```python
from build123d import *

# Parameters (mm, degrees)
ESQUISSE1_W          = 40
ESQUISSE1_H          = 60
PCB_RFID_RC522_DEPTH = 2
ANTENNE_RFID_START   = 2
ESQUISSE2_W          = 30
ESQUISSE2_H          = 32
ESQUISSE2_W_2        = 22
ESQUISSE2_H_2        = 24
ANTENNE_RFID_DEPTH   = 1.2
PUCE_MFRC522_START   = 2
ESQUISSE3_W          = 10
ESQUISSE3_H          = 10
PUCE_MFRC522_DEPTH   = 2.5
ESQUISSE4_W          = 22
ESQUISSE4_H          = 3
CONNECTEUR_SPI_DEPTH = 5


with BuildPart() as part:
    # Esquisse1 → PCB_RFID_RC522 (new body)
    with BuildSketch(Plane.XY):
        Rectangle(ESQUISSE1_W, ESQUISSE1_H)
    extrude(amount=PCB_RFID_RC522_DEPTH)

    # Esquisse2 → Antenne_RFID (add)
    with BuildSketch(Plane.XY.offset(ANTENNE_RFID_START)):
        with Locations((0, 8)):
            Rectangle(ESQUISSE2_W, ESQUISSE2_H)
        with Locations((0, 8)):
            Rectangle(ESQUISSE2_W_2, ESQUISSE2_H_2, mode=Mode.SUBTRACT)
    extrude(amount=ANTENNE_RFID_DEPTH)

    # Esquisse3 → Puce_MFRC522 (add)
    with BuildSketch(Plane.XY.offset(PUCE_MFRC522_START)):
        with Locations((0, -15)):
            Rectangle(ESQUISSE3_W, ESQUISSE3_H)
    extrude(amount=PUCE_MFRC522_DEPTH)

    # Esquisse4 → Connecteur_SPI (add)
    with BuildSketch(Plane.XY):
        with Locations((0, -27.5)):
            Rectangle(ESQUISSE4_W, ESQUISSE4_H)
    extrude(amount=-CONNECTEUR_SPI_DEPTH)


solid = part.part
```
Design review of the part built by this model. Coordinates are the model's own, in mm. A direction names the side the tool comes from. Give positions to 0.01 mm unless a question says otherwise; leave off trailing zeros. Order: outer loops, then holes, each group sorted by start corner. A loop starts at its lowest first (then second) coordinate and runs counter-clockwise, first axis right, second up. Notation, with made-up numbers: (19.5, 73) -> (46.5, 73) arc R31 ccw to (46.5, 104) -> close; hole circle Ø1 at (35, 5.5). An arc over 180 degrees is marked (long way). Write item = value, one per line. Start each with the question number.
(1) For pin 1 (1.5 mm diameter, centred on y = -27.5, z = -2, fed in from +X); pin 2 (0.6 mm diameter, centred on x = -7, z = 3, fed in from +Y); pin 3 (1.2 mm diameter, centred on y = -17, z = 3, fed in from -X), all flat-tipped, find the tip position at first contact; note any pin that passes through.
(2) We need section C-C on z = -2.5. Write out the cut boundary in (x, y).
(3) We need section D-D on x = 8.5. Write out the cut boundary in (y, z).
(4) We need section A-A on y = 9.5. Write out the cut boundary in (x, z), plus the area to 3 significant figures.
(5) To check wall thickness, follow line 1 along X through (y, z) = (-1.5, 2.75); line 2 along Y through (x, z) = (4, -0.5); line 3 along Z through (x, y) = (9, -15). State the ranges of each line that lie inside material, in increasing order.
(6) Mouldability with a two-part tool opening along X and no side actions: class faces 1 (the face through (15, 8, 3)), 2 (the face through (0, -4, 3)), 3 (the face through (0, 8, 2)), 4 (the face through (-15, 8, 3)) as +X half, -X half, draft (parallel to the pull), parting line (faces both ways), or undercut.
(7) We need section B-B on x = 2.5. Write out the cut boundary in (y, z), plus the area to 3 significant figures.
(8) For faces 5 (the face through (-11, 8, 3)), 6 (the face through (-5, -15, 3)), 7 (the face through (-11, -28, -2)), 8 (the face through (0, -29, -2)), list the 3-axis set-ups (+Z, -Z, +X, -X, +Y, -Y) from which the entire face can be reached by the end or side of a thin tool; tool diameter is ignored.
Numbers:
q1.pin_1 = 11
q1.pin_2 = 24
q1.pin_3 = -5
q2.outline = (-11, -29) -> (11, -29) -> (11, -26) -> (-11, -26) -> close
q3.outline = (-30, 0) -> (-29, 0) -> (-29, -5) -> (-26, -5) -> (-26, 0) -> (30, 0) -> (30, 2) -> (24, 2) -> (24, 3.2) -> (20, 3.2) -> (20, 2) -> (-4, 2) -> (-4, 3.2) -> (-8, 3.2) -> (-8, 2) -> (-30, 2) -> close
q4.outline = (-20, 0) -> (20, 0) -> (20, 2) -> (15, 2) -> (15, 3.2) -> (11, 3.2) -> (11, 2) -> (-11, 2) -> (-11, 3.2) -> (-15, 3.2) -> (-15, 2) -> (-20, 2) -> close
q4.area = 89.6 mm^2
q5.line_1 = -15 to -11, 11 to 15
q5.line_2 = -29 to -26
q5.line_3 = 0 to 2
q6.face_1 = +X half
q6.face_2 = undercut
q6.face_3 = undercut
q6.face_4 = -X half
q7.outline = (-30, 0) -> (-29, 0) -> (-29, -5) -> (-26, -5) -> (-26, 0) -> (30, 0) -> (30, 2) -> (24, 2) -> (24, 3.2) -> (20, 3.2) -> (20, 2) -> (-4, 2) -> (-4, 3.2) -> (-8, 3.2) -> (-8, 2) -> (-10, 2) -> (-10, 4.5) -> (-20, 4.5) -> (-20, 2) -> (-30, 2) -> close
q7.area = 170 mm^2
q8.face_5 = +Z
q8.face_6 = +Z, -X, -Y
q8.face_7 = -Z, -X, +Y, -Y
q8.face_8 = -Z, +X, -X, -Y
